from build123d import *

# Parameters (mm, degrees)
SKETCH_1_W          = 15
SKETCH_1_H          = 20
EXTRUDE_1_DEPTH     = 20
SKETCH_5_R          = 5
SKETCH_5_R_2        = 2.75
CUT_EXTRUDE_1_DEPTH = 16
SKETCH_6_R          = 2.75
CUT_EXTRUDE_2_DEPTH = 28.271229432
FILLET_START        = -6
FILLET_2_DEPTH      = 17
CUT_EXTRUDE_4_DEPTH = 0.1
CUT_EXTRUDE_5_DEPTH = 0.1


with BuildPart() as part:
    # Sketch 1 → Extrude 1 (new body)
    with BuildSketch(Plane.XY):
        with Locations((2.694174757, -5.485436893)):
            Rectangle(SKETCH_1_W, SKETCH_1_H)
    extrude(amount=EXTRUDE_1_DEPTH)

    # Sketch 5 → Cut-Extrude 1 (cut)
    with BuildSketch(Plane.XY.offset(20)):
        with Locations((2.701438281, -5.503140696)):
            Circle(SKETCH_5_R)
        with Locations((2.701438281, -5.503140696)):
            Circle(SKETCH_5_R_2, mode=Mode.SUBTRACT)
    extrude(amount=-CUT_EXTRUDE_1_DEPTH, mode=Mode.SUBTRACT)

    # Sketch 6 → Cut-Extrude 2 (cut, through all)
    with BuildSketch(Plane.XY.offset(20)):
        with Locations((2.701438281, -5.503140696)):
            Circle(SKETCH_6_R)
    extrude(amount=-CUT_EXTRUDE_2_DEPTH, mode=Mode.SUBTRACT)

    # Fillet 2: read off the stored shape, not the designer's step
    # Fillet 2 outline → Fillet 2 (cut)
    with BuildSketch(Plane.YZ.offset(FILLET_START)):
        with BuildLine():
            Line((4.514563107, 20), (2.514563107, 20))
            add(Edge.make_bspline(
                [(2.514563107, 20), (4.514563107, 20), (4.514563107, 18)],
                knots=[0, 0, 0, 1, 1, 1], degree=2, weights=[1, 0.707106781, 1]))
            Line((4.514563107, 18), (4.514563107, 20))
        make_face()
        with BuildLine():
            add(Edge.make_bspline(
                [(-13.485436893, 20), (-15.485436893, 20), (-15.485436893, 18)],
                knots=[0, 0, 0, 1, 1, 1], degree=2, weights=[1, 0.707106781, 1]))
            Line((-13.485436893, 20), (-15.485436893, 20))
            Line((-15.485436893, 20), (-15.485436893, 18))
        make_face()
    extrude(amount=FILLET_2_DEPTH, mode=Mode.SUBTRACT)

    # Sketch 7 → Cut-Extrude 4 (cut)
    with BuildSketch(Plane.ZY.offset(4.805825243)):
        with BuildLine():
            Line((0, -15.485436893), (18, -15.485436893))
            ThreePointArc((18, -15.485436893), (19.414213562, -14.899650456), (20, -13.485436893))
            Line((20, -13.485436893), (20, 2.514563107))
            ThreePointArc((20, 2.514563107), (19.414213562, 3.928776669), (18, 4.514563107))
            Line((18, 4.514563107), (0, 4.514563107))
            Line((0, 4.514563107), (0, -15.485436893))
        make_face()
    extrude(amount=-CUT_EXTRUDE_4_DEPTH, mode=Mode.SUBTRACT)

    # Sketch 8 → Cut-Extrude 5 (cut)
    with BuildSketch(Plane(origin=(10.194174757, 0, 0), x_dir=(0, 0, -1), z_dir=(1, 0, 0))):
        with BuildLine():
            Line((-20, 2.514563107), (-20, -13.485436893))
            ThreePointArc((-20, -13.485436893), (-19.414213562, -14.899650456), (-18, -15.485436893))
            Line((-18, -15.485436893), (0, -15.485436893))
            Line((0, -15.485436893), (0, 4.514563107))
            Line((0, 4.514563107), (-18, 4.514563107))
            ThreePointArc((-18, 4.514563107), (-19.414213562, 3.928776669), (-20, 2.514563107))
        make_face()
    extrude(amount=-CUT_EXTRUDE_5_DEPTH, mode=Mode.SUBTRACT)


solid = part.part
Read the model definition and answer for the solid it produces. Units are mm, in the model's axes. A direction names the side the tool comes from. Round coordinates to 2 decimals unless told otherwise and drop trailing zeros. Loops run counter-clockwise (first coordinate to the right, second up) from the corner with the lowest first, then second, coordinate; pieces in that order, holes last.
Q1. Consider probe 1 along X at (y, z) = (-5.5, 14.75); probe 2 along Y at (x, z) = (7, 17); probe 3 along Z at (x, y) = (6, -9). Determine where each line is inside the solid, lowest interval first.
Q2. Section D-D on y = -1.5 is taken. Write down the section's boundary in (x, z), and give its area (3 significant figures).
Q3. This flat-tipped pin is pushed along its axis until it touches: pin 1 (3 mm diameter, centred on x = 1, y = -6, fed in from +Z). Where does it stop, or does it pass through?
Q4. Section B-B on z = 2 is taken. Write down the section's boundary in (x, y).
Q5. Section C-C on y = -7 is taken. Write down the section's boundary in (x, z).
Q6. Section A-A on y = -4 is taken. Write down the section's boundary in (x, z), and give its area (3 significant figures).
Q7. Determine the mould class of faces 3 (the face through (-4.706, -5, 10)), 4 (the face through (-2.3, -3.6, 20)), 5 (the face through (1.618, -10.384, 12.112)), 6 (the face through (10.094, -5, 10)) for opening direction X: released by +X, released by -X, zero draft, split by the parting line, or undercut.
Q8. Which of the six approach directions +Z, -Z, +X, -X, +Y, -Y give full straight-line access (tool end or side, diameter ignored) to faces 1 (the face through (1, -3, 0)), 2 (the face through (5, -8, 4))?
Output:
1. probe 1: x = -4.71 to -2.3, 7.7 to 10.09
1. probe 2: y = -15.49 to -8.06, -2.95 to 4.51
1. probe 3: z = 0 to 4
2. outline: (-4.71, 0) - (10.09, 0) - (10.09, 20) - (5.7, 20) - (5.7, 4) - (-0.29, 4) - (-0.29, 20) - (-4.71, 20) - close
2. area: 200 mm2
3. pin 1: stops at z = 4
4. outline: (-4.71, -15.49) - (10.09, -15.49) - (10.09, 4.51) - (-4.71, 4.51) - close; hole circle Ø5.5 at (2.7, -5.5)
5. outline: (-4.71, 0) - (0.39, 0) - (0.39, 4) - (-2.07, 4) - (-2.07, 20) - (-4.71, 20) - close; (5.01, 0) - (10.09, 0) - (10.09, 20) - (7.47, 20) - (7.47, 4) - (5.01, 4) - close
6. outline: (-4.71, 0) - (0.4, 0) - (0.4, 4) - (-2.07, 4) - (-2.07, 20) - (-4.71, 20) - close; (5, 0) - (10.09, 0) - (10.09, 20) - (7.47, 20) - (7.47, 4) - (5, 4) - close
6. area: 125 mm2
7. face 3: released by -X
7. face 4: zero draft
7. face 5: undercut
7. face 6: released by +X
8. face 1: -Z, +X, -X, +Y, -Y
8. face 2: +Z
